The model under review builds one solid part; all positions refer to its coordinate system, in mm. Face numbers are marked on the shaded views. A direction names the side the tool comes from. Round coordinates to 2 decimals unless told otherwise and drop trailing zeros. Loops run counter-clockwise (first coordinate to the right, second up) from the corner with the lowest first, then second, coordinate; pieces in that order, holes last. Notation, with made-up numbers: M 38,-36 L 80,-36 A12 cw 80,-29 Z; hole C 2,-8.75 d6. An arc over 180 degrees is marked long. Return JSON: item names as keys, results as strings. Group by question number.
Q1. Consider section D-D (y = -3.5). State the section outline as (x, z) points, and give its area (3 significant figures).
Q2. For the marked faces 1 and 2, list the 3-axis set-ups (+Z, -Z, +X, -X, +Y, -Y) from which the entire face can be reached by the end or side of a thin tool; tool diameter is ignored.
Q3. Consider section A-A (y = 0). State the section outline as (x, z) points, and give its area (3 significant figures).
Q4. Draft analysis for pull direction Z (two halves, no side actions). For the marked faces 3, 4 and 5, state which applies: pulls with the +Z half, pulls with the -Z half, needs draft (parallel to the pull), parting line crosses it, or undercut.
Q5. Clearance check with flat-ended pins moving along their axes: pin 1 Ø1 at (y, z) = (-3, 14.5) entering from -X; pin 2 Ø12 at (x, z) = (18, 19) entering from -Y; pin 3 Ø4 at (y, z) = (1, 52.5) entering from -X. State where each tip first meets the part, or that it passes through.
Q6. To check wall thickness, follow line 1 along X through (y, z) = (-6.75, 21.5); line 2 along Z through (x, y) = (-26.5, -8.25); line 3 along Z through (x, y) = (-26.5, 8). State the ranges of each line that lie inside material, in increasing order.
Q7. Consider section B-B (z = 28.5). State the section outline as (x, y) points.
Q8. Consider section C-C (x = -8). State the section outline as (y, z) points.
from build123d import *

# Parameters (mm, degrees)
SKETCH1_R           = 10
BOSS_EXTRUDE1_DEPTH = 60
SKETCH2_R           = 12
BOSS_EXTRUDE2_DEPTH = 2
BOSS_EXTRUDE3_START = 2
SKETCH3_R           = 12
BOSS_EXTRUDE3_DEPTH = 2
SKETCH4_R           = 10
BOSS_EXTRUDE4_DEPTH = 30
SKETCH5_R           = 12
BOSS_EXTRUDE5_DEPTH = 2
BOSS_EXTRUDE6_START = 2
SKETCH6_R           = 12
BOSS_EXTRUDE6_DEPTH = 2


with BuildPart() as part:
    # Sketch1 → Boss-Extrude1 (new body)
    with BuildSketch(Plane.XY):
        Circle(SKETCH1_R)
    extrude(amount=BOSS_EXTRUDE1_DEPTH)

    # Sketch2 → Boss-Extrude2 (add)
    with BuildSketch(Plane.XY.offset(60)):
        Circle(SKETCH2_R)
    extrude(amount=BOSS_EXTRUDE2_DEPTH)

    # Sketch3 → Boss-Extrude3 (add)
    with BuildSketch(Plane(origin=(0, 0, 0), x_dir=(-1, 0, 0), z_dir=(0, 0, -1)).offset(BOSS_EXTRUDE3_START)):
        with Locations(Location((0, 0, 0), (0, 0, 180))):
            Circle(SKETCH3_R)
    extrude(amount=-BOSS_EXTRUDE3_DEPTH)

    # Sketch4 → Boss-Extrude4 (add, symmetric)
    with BuildSketch(Plane(origin=(0, 0, 0), x_dir=(0, 0, -1), z_dir=(1, 0, 0))):
        with Locations(Location((-30.27140407, 0, 0), (0, 0, 270))):
            Circle(SKETCH4_R)
    extrude(amount=BOSS_EXTRUDE4_DEPTH, both=True)

    # Sketch5 → Boss-Extrude5 (add)
    with BuildSketch(Plane(origin=(30, 0, 0), x_dir=(0, 0, -1), z_dir=(1, 0, 0))):
        with Locations((-30.27140407, 0)):
            Circle(SKETCH5_R)
    extrude(amount=BOSS_EXTRUDE5_DEPTH)

    # Sketch6 → Boss-Extrude6 (add)
    with BuildSketch(Plane.ZY.offset(30).offset(BOSS_EXTRUDE6_START)):
        with Locations(Location((30.27140407, 0, 0), (0, 0, 180))):
            Circle(SKETCH6_R)
    extrude(amount=-BOSS_EXTRUDE6_DEPTH)


solid = part.part
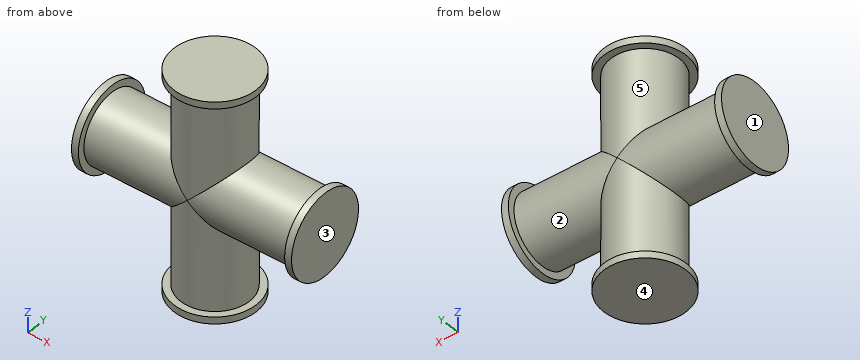
Values:
{
 "1": {"outline": "M -32,18.79 L -30,18.79 L -30,20.9 L -9.37,20.9 L -9.37,0 L -11.48,0 L -11.48,-2 L 11.48,-2 L 11.48,0 L 9.37,0 L 9.37,20.9 L 30,20.9 L 30,18.79 L 32,18.79 L 32,41.75 L 30,41.75 L 30,39.64 L 9.37,39.64 L 9.37,60 L 11.48,60 L 11.48,62 L -11.48,62 L -11.48,60 L -9.37,60 L -9.37,39.64 L -30,39.64 L -30,41.75 L -32,41.75 Z", "area": "2,080 mm2"},
 "2": {"face 1": "+Z, -Z, -X, +Y, -Y", "face 2": "none"},
 "3": {"outline": "M -32,18.27 L -30,18.27 L -30,20.27 L -10,20.27 L -10,0 L -12,0 L -12,-2 L 12,-2 L 12,0 L 10,0 L 10,20.27 L 30,20.27 L 30,18.27 L 32,18.27 L 32,42.27 L 30,42.27 L 30,40.27 L 10,40.27 L 10,60 L 12,60 L 12,62 L -12,62 L -12,60 L -10,60 L -10,40.27 L -30,40.27 L -30,42.27 L -32,42.27 Z", "area": "2,190 mm2"},
 "4": {"face 3": "needs draft", "face 4": "pulls with the -Z half", "face 5": "undercut"},
 "5": {"pin 1": "stops at x = -9.68", "pin 2": "stops at y = -8.5", "pin 3": "stops at x = -10"},
 "6": {"line 1": "x = -32 to -30, -7.38 to 7.38, 30 to 32", "line 2": "z = 24.62 to 35.92", "line 3": "z = 24.27 to 36.27"},
 "7": {"outline": "M -32,-11.87 L -30,-11.87 L -30,-9.84 L -1.77,-9.84 A10 ccw 1.77,-9.84 L 30,-9.84 L 30,-11.87 L 32,-11.87 L 32,11.87 L 30,11.87 L 30,9.84 L 1.77,9.84 A10 ccw -1.77,9.84 L -30,9.84 L -30,11.87 L -32,11.87 Z"},
 "8": {"outline": "M -8.94,-2 L 8.94,-2 L 8.94,0 L 6,0 L 6,22.27 A10 ccw 6,38.27 L 6,60 L 8.94,60 L 8.94,62 L -8.94,62 L -8.94,60 L -6,60 L -6,38.27 A10 ccw -6,22.27 L -6,0 L -8.94,0 Z"}
}
